Source: CAD feature listing. Evaluate the final solid. Frame: model axes, mm. A direction names the side the tool comes from. Coordinates: 2 decimals unless noted, no trailing zeros. Loops run counter-clockwise (first coordinate to the right, second up) from the corner with the lowest first, then second, coordinate; pieces in that order, holes last.
Item 1: Section query A-A, the plane y = 36. Return the cut outline in (x, z).
Item 2: Line query: probe 1 along Y at (x, z) = (10.55, 0); probe 2 along Z at (x, y) = (8, -10.5); probe 3 along Y at (x, z) = (4.25, 17). Output: solid intervals per line, ascending.
Item 3: Section query D-D, the plane y = -66. Return the cut outline in (x, z).
Item 4: Section query B-B, the plane z = 28.5. Return the cut outline in (x, y).
Item 5: Pull-direction query (Y, two-part tool) for faces 4 (the flat face through (3, -80.5, -15)), 5 (the cylindrical face through (5.92, 56.99, -38.65)), 6 (the flat face through (6, -171, 6)); classes: +Y half, -Y half, draft (parallel to the pull), parting line (faces both ways), or undercut.
Item 6: Pin query (flat end, axial travel): pin 1 Ø1 at (x, y) = (10, -108) entering from +Z; pin 2 Ø1.2 at (x, z) = (3, 37.5) entering from -Y. Return the tip coordinate at first contact, or that it passes through.
Item 7: Reachability of faces 1 (the flat face through (8, -78, -7)), 2 (the flat face through (6.5, -147, 28)), 3 (the flat face through (3, -75.5, -14)) from +Z, -Z, +X, -X, +Y, -Y: full face, straight path, thin tool, end or side. Return the list, or none.
Item 8: Section query C-C, the plane y = -147. Return the cut outline in (x, z), then the cut area to 4 significant figures.
```python
from build123d import *

# Parameters (mm, degrees)
SKETCH1_W                          = 63
SKETCH1_H                          = 120
SKETCH1_R                          = 20
BOSS_EXTRUDE1_DEPTH                = 12
F_5_0_5_DIAMETER_HOLE2_D           = 5
LINEAR_RAIL_MOUNT_HOLE_D           = 5
LINEAR_RAIL_MOUNT_HOLE_CBORE_D     = 12
LINEAR_RAIL_MOUNT_HOLE_CBORE_DEPTH = 6
BOSS_EXTRUDE2_DEPTH                = 12
SKETCH9_W                          = 52
SKETCH9_H                          = 111
BOSS_EXTRUDE3_DEPTH                = 12
SKETCH11_W                         = 10
SKETCH11_H                         = 160
BOSS_EXTRUDE4_DEPTH                = 12
F_5_0_5_DIAMETER_HOLE1_D           = 5
FILLET1_R                          = 10
CUT_EXTRUDE1_REACH                 = 181.876
CUT_EXTRUDE2_DEPTH                 = 8
CUT_EXTRUDE3_DEPTH                 = 6.5
LPATTERN1_COUNT                    = 2
LPATTERN1_PITCH                    = 69
MIRROR1_COPY_1_DEPTH               = 8
MIRROR1_COPY_2_DEPTH               = 6.5


with BuildPart() as part:
    # Sketch1 → Boss-Extrude1 (new body)
    with BuildSketch(Plane(origin=(0, 0, 0), x_dir=(0, 0, -1), z_dir=(1, 0, 0))):
        Rectangle(SKETCH1_W, SKETCH1_H)
        Circle(SKETCH1_R, mode=Mode.SUBTRACT)
    extrude(amount=BOSS_EXTRUDE1_DEPTH)

    # Ø5.0 (5) Diameter Hole2 (through all)
    with Locations(Plane.ZY):
        with Locations((-23.5, 23.5), (23.5, 23.5), (23.5, -23.5), (-23.5, -23.5)):
            Hole(F_5_0_5_DIAMETER_HOLE2_D / 2)

    # Linear Rail Mount Hole (through all)
    with Locations(Plane.ZY):
        with Locations((0, 45), (0, -45)):
            CounterBoreHole(LINEAR_RAIL_MOUNT_HOLE_D / 2, LINEAR_RAIL_MOUNT_HOLE_CBORE_D / 2, LINEAR_RAIL_MOUNT_HOLE_CBORE_DEPTH)

    # Sketch8 → Boss-Extrude2 (add)
    with BuildSketch(Plane.ZY):
        Polygon((44.5, 18), (44.5, -12), (54.5, -12), (54.5, 60), (31.5, 60), (31.5, -60), (32.5, -60), (32.5, 18), align=None)
    extrude(amount=-BOSS_EXTRUDE2_DEPTH)

    # Sketch9 → Boss-Extrude3 (add)
    with BuildSketch(Plane.ZY):
        with Locations((6.5, -115.5)):
            Rectangle(SKETCH9_W, SKETCH9_H)
    extrude(amount=-BOSS_EXTRUDE3_DEPTH)

    # Sketch11 → Boss-Extrude4 (add)
    with BuildSketch(Plane(origin=(12, 0, 0), x_dir=(0, 0, -1), z_dir=(1, 0, 0))):
        with Locations((36.5, -20)):
            Rectangle(SKETCH11_W, SKETCH11_H)
    extrude(amount=-BOSS_EXTRUDE4_DEPTH)

    # Ø5.0 (5) Diameter Hole1 (through all)
    with Locations(Plane(origin=(12, 0, 0), x_dir=(0, 0, -1), z_dir=(1, 0, 0))):
        with Locations((-36.5, 36)):
            Hole(F_5_0_5_DIAMETER_HOLE1_D / 2)

    # Fillet1
    fillet1_edges = [part.edges().sort_by_distance(p)[0] for p in [
        (6, 60, 54.5),
        (6, -12, 54.5),
        (6, -100, -41.5),
        (6, 60, -41.5),
    ]]
    fillet(fillet1_edges, radius=FILLET1_R - 0.0001)  # a hair under: the kernel refuses the full size

    # Sketch25 → Cut-Extrude1 (cut, up to next)
    with BuildSketch(Plane.ZY, mode=Mode.PRIVATE) as cut_extrude1_sk1:
        with BuildLine():
            Line((32.5, 18), (36.5, 18))
            ThreePointArc((36.5, 18), (34.5, 20), (32.5, 18))
        make_face()
    cut_extrude1_tool1 = extrude(cut_extrude1_sk1.sketch, amount=-CUT_EXTRUDE1_REACH, mode=Mode.PRIVATE) & part.part
    # Sketch25 → Cut-Extrude1 (cut, up to next)
    with BuildSketch(Plane.ZY, mode=Mode.PRIVATE) as cut_extrude1_sk2:
        with BuildLine():
            Line((40.5, 18), (44.5, 18))
            ThreePointArc((44.5, 18), (42.5, 20), (40.5, 18))
        make_face()
    cut_extrude1_tool2 = extrude(cut_extrude1_sk2.sketch, amount=-CUT_EXTRUDE1_REACH, mode=Mode.PRIVATE) & part.part
    # Sketch25 → Cut-Extrude1 (cut, up to next)
    with BuildSketch(Plane.ZY, mode=Mode.PRIVATE) as cut_extrude1_sk3:
        with BuildLine():
            Line((-31.5, -60), (-27.5, -60))
            ThreePointArc((-27.5, -60), (-29.5, -58), (-31.5, -60))
        make_face()
    cut_extrude1_tool3 = extrude(cut_extrude1_sk3.sketch, amount=-CUT_EXTRUDE1_REACH, mode=Mode.PRIVATE) & part.part
    # Sketch25 → Cut-Extrude1 (cut, up to next)
    with BuildSketch(Plane.ZY, mode=Mode.PRIVATE) as cut_extrude1_sk4:
        with BuildLine():
            Line((-23.5, -60), (-19.5, -60))
            ThreePointArc((-19.5, -60), (-21.5, -58), (-23.5, -60))
        make_face()
    cut_extrude1_tool4 = extrude(cut_extrude1_sk4.sketch, amount=-CUT_EXTRUDE1_REACH, mode=Mode.PRIVATE) & part.part
    add(cut_extrude1_tool1.solids().sort_by_distance((0, 18.848826, 34.5))[0], mode=Mode.SUBTRACT)
    add(cut_extrude1_tool2.solids().sort_by_distance((0, 18.848826, 42.5))[0], mode=Mode.SUBTRACT)
    add(cut_extrude1_tool3.solids().sort_by_distance((0, -59.151174, -29.5))[0], mode=Mode.SUBTRACT)
    add(cut_extrude1_tool4.solids().sort_by_distance((0, -59.151174, -21.5))[0], mode=Mode.SUBTRACT)

    # Sketch27 → Cut-Extrude2 (cut)
    with BuildSketch(Plane(origin=(0, 35.243272034, 16.659279863), x_dir=(0, 0, 1), z_dir=(-1, 0, 0))):
        with BuildLine():
            Line((5.840720137, -178.243272034), (5.840720137, -186.243272034))
            ThreePointArc((5.840720137, -186.243272034), (3.840720137, -188.243272034), (1.840720137, -186.243272034))
            Line((1.840720137, -186.243272034), (1.840720137, -178.243272034))
            ThreePointArc((1.840720137, -178.243272034), (3.840720137, -176.243272034), (5.840720137, -178.243272034))
        make_face()
    cut_extrude2 = extrude(amount=-CUT_EXTRUDE2_DEPTH, mode=Mode.SUBTRACT)

    # Sketch29 → Cut-Extrude3 (cut)
    with BuildSketch(Plane(origin=(0, 35.243272034, 16.659279863), x_dir=(0, 0, 1), z_dir=(-1, 0, 0))):
        with BuildLine():
            Line((61.738206335, -184.743272034), (-1.159279863, -184.743272034))
            ThreePointArc((-1.159279863, -184.743272034), (-3.659279863, -182.243272034), (-1.159279863, -179.743272034))
            Line((-1.159279863, -179.743272034), (61.738206335, -179.743272034))
            ThreePointArc((61.738206335, -179.743272034), (64.238206335, -182.243272034), (61.738206335, -184.743272034))
        make_face()
    cut_extrude3 = extrude(amount=-CUT_EXTRUDE3_DEPTH, mode=Mode.SUBTRACT)

    # LPattern1: Cut-Extrude2, Cut-Extrude3 ×2
    with Locations(*[(0, i * LPATTERN1_PITCH, 0) for i in range(1, LPATTERN1_COUNT)]):
        add(cut_extrude2, mode=Mode.SUBTRACT)
        add(cut_extrude3, mode=Mode.SUBTRACT)

    # Mirror1: Cut-Extrude2, Cut-Extrude3 across plane
    add(cut_extrude2.mirror(Plane.XY.offset(6.5)), mode=Mode.SUBTRACT)
    add(cut_extrude3.mirror(Plane.XY.offset(6.5)), mode=Mode.SUBTRACT)

    # Mirror1 copy 1 sketch → Mirror1 copy 1 (cut)
    with BuildSketch(Plane(origin=(0, 104.243272034, -3.659279863), x_dir=(0, 0, -1), z_dir=(-1, 0, 0))):
        with BuildLine():
            Line((5.840720137, 178.243272034), (5.840720137, 186.243272034))
            ThreePointArc((5.840720137, 186.243272034), (3.840720137, 188.243272034), (1.840720137, 186.243272034))
            Line((1.840720137, 186.243272034), (1.840720137, 178.243272034))
            ThreePointArc((1.840720137, 178.243272034), (3.840720137, 176.243272034), (5.840720137, 178.243272034))
        make_face()
    extrude(amount=-MIRROR1_COPY_1_DEPTH, mode=Mode.SUBTRACT)

    # Mirror1 copy 2 sketch → Mirror1 copy 2 (cut)
    with BuildSketch(Plane(origin=(0, 104.243272034, -3.659279863), x_dir=(0, 0, -1), z_dir=(-1, 0, 0))):
        with BuildLine():
            Line((61.738206335, 184.743272034), (-1.159279863, 184.743272034))
            ThreePointArc((-1.159279863, 184.743272034), (-3.659279863, 182.243272034), (-1.159279863, 179.743272034))
            Line((-1.159279863, 179.743272034), (61.738206335, 179.743272034))
            ThreePointArc((61.738206335, 179.743272034), (64.238206335, 182.243272034), (61.738206335, 184.743272034))
        make_face()
    extrude(amount=-MIRROR1_COPY_2_DEPTH, mode=Mode.SUBTRACT)


solid = part.part
```
Verdict:
1. outline: (0, -41.5) - (12, -41.5) - (12, 34) - (0, 34) - close; (0, 39) - (12, 39) - (12, 54.5) - (0, 54.5) - close
2. probe 1: y = -171 to -47.5, -42.5 to -20, 20 to 42.5, 47.5 to 60
2. probe 2: z = -41.5 to -17.02, 17.02 to 32.5, 44.5 to 49.77
2. probe 3: y = -171 to -149.5, -144.5 to -80.5, -75.5 to -10.54, 10.54 to 60
3. outline: (0, -41.5) - (12, -41.5) - (12, -31.5) - (0, -31.5) - close; (0, -19.5) - (12, -19.5) - (12, 32.5) - (0, 32.5) - close
4. outline: (0, -171) - (12, -171) - (12, 60) - (0, 60) - (0, -75.5) - (6.5, -75.5) - (6.5, -80.5) - (0, -80.5) - (0, -144.5) - (6.5, -144.5) - (6.5, -149.5) - (0, -149.5) - close
5. face 4: undercut
5. face 5: +Y half
5. face 6: -Y half
6. pin 1: stops at z = 32.5
6. pin 2: stops at y = 18
7. face 1: -X
7. face 2: +Z, -X
7. face 3: -Z, -X
8. outline: (0, 0) - (6.5, 0) - (6.5, -5.5) - (8, -5.5) - (8, -9.5) - (6.5, -9.5) - (6.5, -19.5) - (12, -19.5) - (12, 32.5) - (6.5, 32.5) - (6.5, 22.5) - (8, 22.5) - (8, 18.5) - (6.5, 18.5) - (6.5, 13) - (0, 13) - close
8. area: 358.5 mm2
